from build123d import *

# Parameters (mm, degrees)
SKETCH1_R           = 14.2875
SKETCH1_R_2         = 9.525
SKETCH1_R_3         = 2.54
BOSS_EXTRUDE1_DEPTH = 19.05
FILLET1_R           = 4.7625


with BuildPart() as part:
    # Sketch1 → Boss-Extrude1 (new body)
    with BuildSketch(Plane(origin=(0, 0, 0), x_dir=(0, 0, -1), z_dir=(1, 0, 0))):
        with BuildLine():
            Line((54.102, 134.9375), (0, 134.9375))
            Line((0, 134.9375), (0, 255.983795331))
            ThreePointArc((0, 255.983795331), (11.524561047, 292.463978248), (41.915078603, 315.702646361))
            add(Edge.make_bspline(
                [(685.8, 211.1375), (685.8, 548.429920531), (41.915078603, 315.702646361)],
                knots=[0, 0, 0, 2.332266964, 2.332266964, 2.332266964], degree=2, weights=[1, 0.393708858, 1]))
            Line((685.8, 211.1375), (685.8, 134.9375))
            Line((685.8, 134.9375), (631.698, 134.9375))
            Line((631.698, 134.9375), (631.698, 107.95))
            Line((631.698, 107.95), (463.55, 107.95))
            Line((463.55, 107.95), (463.55, 171.45))
            Line((463.55, 171.45), (238.76, 171.45))
            Line((238.76, 171.45), (238.76, 77.7875))
            Line((238.76, 77.7875), (54.102, 77.7875))
            Line((54.102, 77.7875), (54.102, 134.9375))
        make_face()
        with Locations(Location((25.4, 234.95, 0), (0, 0, 180))):
            Circle(SKETCH1_R, mode=Mode.SUBTRACT)
        with Locations(Location((50.8, 272.96523905, 0), (0, 0, 180))):
            Circle(SKETCH1_R_2, mode=Mode.SUBTRACT)
        with Locations(Location((73.66, 282.447875814, 0), (0, 0, 180))):
            Circle(SKETCH1_R_3, mode=Mode.SUBTRACT)
        with Locations(Location((27.94, 263.482602286, 0), (0, 0, 180))):
            Circle(SKETCH1_R_3, mode=Mode.SUBTRACT)
        with Locations(Location((76.372962562, 257.848285692, 0), (0, 0, 180))):
            Circle(SKETCH1_R_2, mode=Mode.SUBTRACT)
        with Locations(Location((79.085925124, 233.248695571, 0), (0, 0, 180))):
            Circle(SKETCH1_R_3, mode=Mode.SUBTRACT)
    extrude(amount=BOSS_EXTRUDE1_DEPTH)

    # Fillet1
    fillet1_edges = [part.edges().sort_by_distance(p)[0] for p in [
        (9.525, 134.9375, -631.698),
        (9.525, 171.45, -463.55),
        (9.525, 171.45, -238.76),
        (9.525, 134.9375, -54.102),
    ]]
    fillet(fillet1_edges, radius=FILLET1_R)


solid = part.part
Source: CAD feature listing. Evaluate the final solid. Frame: model axes, mm. A direction names the side the tool comes from. Round coordinates to 2 decimals unless told otherwise and drop trailing zeros. Use a Markdown table: item, result. Add a question column.
1. Mould query, pull axis Z, two halves, no side actions, for faces 1 (the cylindrical face through (9.39, 263.52, -52.04)), 2 (the flat face through (9, 134.938, -661)), 3 (the flat face through (9, 171.45, -353)), 4 (the flat face through (9, 195, 0)). Classes: +Z half, -Z half, draft (parallel to the pull), parting line (faces both ways), or undercut.
2. Line query: probe 1 along Y at (x, z) = (15.25, -73.66); probe 2 along Z at (x, y) = (11.5, 166); probe 3 along Z at (x, y) = (1, 98). Output: solid intervals per line, ascending.
3. First-contact query: pin 1 (5.5 mm diameter, centred on x = 10.5, z = -556, fed in from -Y); pin 2 (3 mm diameter, centred on x = 16.5, y = 226.5, fed in from -Z); pin 3 (5.5 mm diameter, centred on x = 11.5, z = -373.5, fed in from -Y). Flat tips, straight axial feed; report the tip coordinate or a pass-through.
4. Section query A-A (x = 15.25). Give the number of separate pieces and of enclosed holes in the cut face, then the cut area to 3 significant figures.
5. Set-up query: faces 5 (the flat face through (0, 212, -348)), 6 (the flat face through (9, 123, -238.76)), 7 (the flat face through (9, 119, -631.698)), 8 (the flat face through (9, 134.938, -25)). Return all of +Z, -Z, +X, -X, +Y, -Y with unobstructed straight access to the full face (end or side cutting, diameter ignored); none if empty.
Derived:
| question | item | result |
|---|---|---|
| 1 | face 1 | undercut |
| 1 | face 2 | draft |
| 1 | face 3 | undercut |
| 1 | face 4 | +Z half |
| 2 | probe 1 | 77.79 to 248.72, 266.98 to 279.91, 284.99 to 325.98 |
| 2 | probe 2 | -685.8 to -463.55, -238.76 to 0 |
| 2 | probe 3 | -238.76 to -54.1 |
| 3 | pin 1 | y = 107.95 |
| 3 | pin 2 | z = -684.04 |
| 3 | pin 3 | y = 171.45 |
| 4 | separate pieces | 1 |
| 4 | enclosed holes | 6 |
| 4 | area | 140,000 mm2 |
| 5 | face 5 | +Z, -Z, -X, +Y, -Y |
| 5 | face 6 | +X, -X, -Y |
| 5 | face 7 | -Z, +X, -X, -Y |
| 5 | face 8 | +Z, +X, -X, -Y |
